For this review, take the finished solid that the model builds, in its own axes (mm). A direction names the side the tool comes from. Round coordinates to 2 decimals unless told otherwise and drop trailing zeros. Order: outer loops, then holes, each group sorted by start corner. A loop starts at its lowest first (then second) coordinate and runs counter-clockwise, first axis right, second up. Notation, with made-up numbers: M -31.75,10.25 L -24.75,10.25 A20 cw -24.75,44.25 Z; hole C 39.5,60.5 d2. An arc over 180 degrees is marked long. Answer as a JSON object with one key per item and string values.
from build123d import *

# Parameters (mm, degrees)
F0_W     = 42
F0_H     = 13
F1_DEPTH = 13
F2_R     = 1
F3_DEPTH = 12
F4_R     = 1.5
F5_DEPTH = 13.001


with BuildPart() as f1:
    # F0 (on Top) → F1 (new body)
    with BuildSketch(Plane.XY):
        Rectangle(F0_W, F0_H)
    extrude(amount=F1_DEPTH)

    # F2 (on face) → F3 (cut)
    with BuildSketch(Plane.XY.offset(13)):
        with Locations((-16.753747, 1)):
            Circle(F2_R)
        with Locations((-5.253747, -1)):
            Circle(F2_R)
        with Locations((5.253747, -1)):
            Circle(F2_R)
        with Locations((16.753747, 1)):
            Circle(F2_R)
    extrude(amount=-F3_DEPTH, mode=Mode.SUBTRACT)

    # F4 (on face) → F5 (cut, through all)
    with BuildSketch(Plane.XY.offset(13)):
        Circle(F4_R)
    extrude(amount=-F5_DEPTH, mode=Mode.SUBTRACT)


solid = f1.part
1) Add section B-B on z = 6.5. State the section outline as (x, y) points, and give its area (3 significant figures).
Geometry check:
{"outline": "M -21,-6.5 L 21,-6.5 L 21,6.5 L -21,6.5 Z; hole C -16.75,1 d2; hole C -5.25,-1 d2; hole C 0,0 d3; hole C 5.25,-1 d2; hole C 16.75,1 d2", "area": "526 mm²"}
2) Mouldability with a two-part tool opening along Y and no side actions: class faces 3 (the flat face through (-5, -1, 1)), 4 (the flat face through (21, 0, 6)), 5 (the flat face through (0, 6.5, 6)) as +Y half, -Y half, draft (parallel to the pull), parting line (faces both ways), or undercut.
Geometry check:
{"face 3": "undercut", "face 4": "draft", "face 5": "+Y half"}
3) Add section D-D on x = 5. State the section outline as (y, z) points.
Geometry check:
{"outline": "M -6.5,0 L 6.5,0 L 6.5,13 L -0.03,13 L -0.03,1 L -1.97,1 L -1.97,13 L -6.5,13 Z"}
4) Insertion check: P1, Ø1.2, axis at x = 5.25, y = -1, coming from the +Z side. The pin has a flat end and moves straight along its axis. Give the tip position at first contact, or say it passes through.
Geometry check:
{"P1": "stops at z = 1"}
5) For L1, parallel to X at y = -0.75, z = 2; L2, parallel to Y at x = 16, z = 4.5; L3, parallel to Z at x = -17.5, y = 1.25, list the stretches that pass through material, from the lowest coordinate up.
Geometry check:
{"L1": "x = -21 to -6.22, -4.29 to -1.3, 1.3 to 4.29, 6.22 to 21", "L2": "y = -6.5 to 0.34, 1.66 to 6.5", "L3": "z = 0 to 1"}
6) Machinability: for faces 1 (the flat face through (0, -6.5, 6)), 2 (the cylindrical face through (-15.8, 1.3, 7.1)), which of the approach directions +Z, -Z, +X, -X, +Y, -Y give a long, thin tool a straight path to every point of the face, cutting with its end or side? Answer none if there is none.
Geometry check:
{"face 1": "+Z, -Z, +X, -X, -Y", "face 2": "+Z"}
7) Add section C-C on y = 1. State the section outline as (x, z) points, and give its area (3 significant figures).
Geometry check:
{"outline": "M -21,0 L -1.12,0 L -1.12,13 L -15.75,13 L -15.75,1 L -17.75,1 L -17.75,13 L -21,13 Z; M 1.12,0 L 21,0 L 21,13 L 17.75,13 L 17.75,1 L 15.75,1 L 15.75,13 L 1.12,13 Z", "area": "469 mm²"}
8) Add section A-A on x = 0. State the section outline as (y, z) points, and give its area (3 significant figures).
Geometry check:
{"outline": "M -6.5,0 L -1.5,0 L -1.5,13 L -6.5,13 Z; M 1.5,0 L 6.5,0 L 6.5,13 L 1.5,13 Z", "area": "130 mm²"}
